```python
from build123d import *
from build123d.topology import SkipClean

# Parameters (mm, degrees)
BOSS_EXTRUDE1_DEPTH = 5
SKETCH2_R           = 2.6
SKETCH2_R_2         = 1.6
EXTRUDE_THIN1_DEPTH = 1


with BuildPart() as part:
    # Sketch1 → Boss-Extrude1 (new body)
    with BuildSketch(Plane(origin=(0, 0, 0), x_dir=(0, 0, -1), z_dir=(1, 0, 0))):
        with BuildLine():
            Line((15, 30), (7.5, 30))
            Line((7.5, 30), (7.5, 21.6))
            ThreePointArc((7.5, 21.6), (8.63137085, 21.13137085), (9.1, 20))
            ThreePointArc((9.1, 20), (8.63137085, 18.86862915), (7.5, 18.4))
            Line((7.5, 18.4), (7.5, 9.1))
            ThreePointArc((7.5, 9.1), (8.63137085, 8.63137085), (9.1, 7.5))
            ThreePointArc((9.1, 7.5), (8.63137085, 6.36862915), (7.5, 5.9))
            Line((7.5, 5.9), (7.5, 0))
            Line((7.5, 0), (15, 0))
            Line((15, 0), (15, 30))
        make_face()
        with BuildLine():
            Line((7.5, 21.6), (7.5, 30))
            Line((7.5, 30), (0, 30))
            Line((0, 30), (0, 0))
            Line((0, 0), (7.5, 0))
            Line((7.5, 0), (7.5, 5.9))
            ThreePointArc((7.5, 5.9), (5.9, 7.5), (7.5, 9.1))
            Line((7.5, 9.1), (7.5, 18.4))
            ThreePointArc((7.5, 18.4), (5.9, 20), (7.5, 21.6))
        make_face()
    extrude(amount=BOSS_EXTRUDE1_DEPTH)

    # Sketch2 → Extrude-Thin1 (add)
    with SkipClean():  # the faces are left unmerged after this step: merging them gives an invalid solid
        with BuildSketch(Plane(origin=(5, 0, 0), x_dir=(0, 0, -1), z_dir=(1, 0, 0))):
            with Locations((7.5, 7.5)):
                Circle(SKETCH2_R)
            with Locations((7.5, 7.5)):
                Circle(SKETCH2_R_2, mode=Mode.SUBTRACT)
        extrude(amount=EXTRUDE_THIN1_DEPTH)


solid = part.part
```
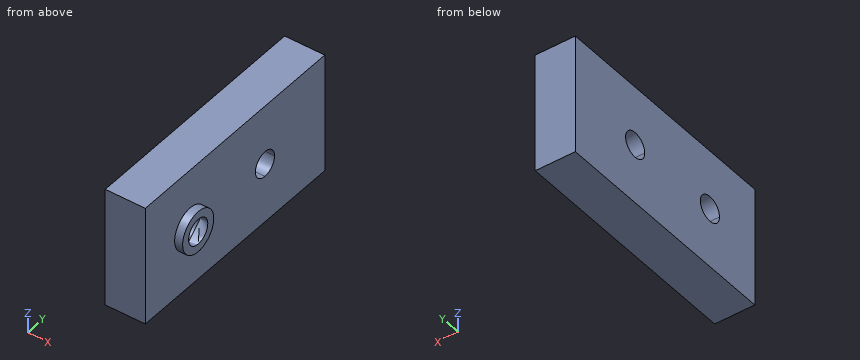
Source: CAD feature listing. Evaluate the final solid. Frame: model axes, mm. Coordinates: 2 decimals unless noted, no trailing zeros. Loops run counter-clockwise (first coordinate to the right, second up) from the corner with the lowest first, then second, coordinate; pieces in that order, holes last. Notation, with made-up numbers: (-16.75, 84) -> (26.25, 84) arc R24 ccw to (26.25, 107) -> close; hole circle Ø9 at (76.5, 77). An arc over 180 degrees is marked (long way). One line per item, written item: value. Start each with the question number.
Q1. Section query D-D, the plane z = -4. Return the cut outline in (x, y), and give its area (3 significant figures).
Q2. Section query C-C, the plane y = 3.75. Return the cut outline in (x, z).
Q3. Line query: line 1 along Y through (x, z) = (5.7, -7.5); line 2 along X through (y, z) = (10, -3.75); line 3 along Z through (x, y) = (4.45, 8.5). Output: solid intervals per line, ascending.
Q4. Section query A-A, the plane x = 3. Return the cut outline in (y, z), and give its area (3 significant figures).
Q5. Section query B-B, the plane z = -7. Return the cut outline in (x, y).
Results:
1. outline: (0, 0) -> (5, 0) -> (5, 30) -> (0, 30) -> close
1. area: 150 mm^2
2. outline: (0, -15) -> (5, -15) -> (5, 0) -> (0, 0) -> close
3. line 1: 4.9 to 5.9, 9.1 to 10.1
3. line 2: 0 to 5
3. line 3: -15 to -8.75, -6.25 to 0
4. outline: (0, -15) -> (30, -15) -> (30, 0) -> (0, 0) -> close; hole circle Ø3.2 at (7.5, -7.5); hole circle Ø3.2 at (20, -7.5)
4. area: 434 mm^2
5. outline: (0, 0) -> (5, 0) -> (5, 4.95) -> (6, 4.95) -> (6, 5.98) -> (0, 5.98) -> close; (0, 9.02) -> (6, 9.02) -> (6, 10.05) -> (5, 10.05) -> (5, 18.48) -> (0, 18.48) -> close; (0, 21.52) -> (5, 21.52) -> (5, 30) -> (0, 30) -> close
